Part print with two shaded views. Sizes in mm from the minimum x, y, z corner. A direction names the side the tool comes from. Coordinates: 2 decimals unless noted, no trailing zeros. Loops run counter-clockwise (first coordinate to the right, second up) from the corner with the lowest first, then second, coordinate; pieces in that order, holes last.
(1) Slice it at C-C (x = 3.5). Give the cut face in (y, z).
(2) Two-plate mould, pull along X, no slides. Class the marked faces 3, 4 and 5: pulls with the +X half, pulls with the -X half, needs draft (parallel to the pull), parting line crosses it, or undercut.
(3) Flat gauge pins, fed straight in: P1, Ø0.9, axis at x = 46, y = 36.5, coming from the +Z side; P2, Ø11.5, axis at x = 26.5, y = 22, coming from the +Z side. Where does each tip first touch, or does it go through?
(4) Slice it at A-A (z = 11.25). Give the cut face in (x, y), and give its area (3 significant figures).
(5) Slice it at D-D (z = 7.75). Give the cut face in (x, y).
(6) Tool access for the marked faces 1 and 2: list every direction of +Z, -Z, +X, -X, +Y, -Y with a clear straight run to the whole face (end or side of a thin tool).
(7) Wall check: L1, parallel to Y at x = 46.5, z = 15; L2, parallel to X at y = 2.5, z = 1.25; L3, parallel to Y at x = 43.5, z = 7.25. Give the ranges that are in metal, low to high.
(8) Slice it at B-B (y = 22). Give the cut face in (x, z), and give its area (3 significant figures).
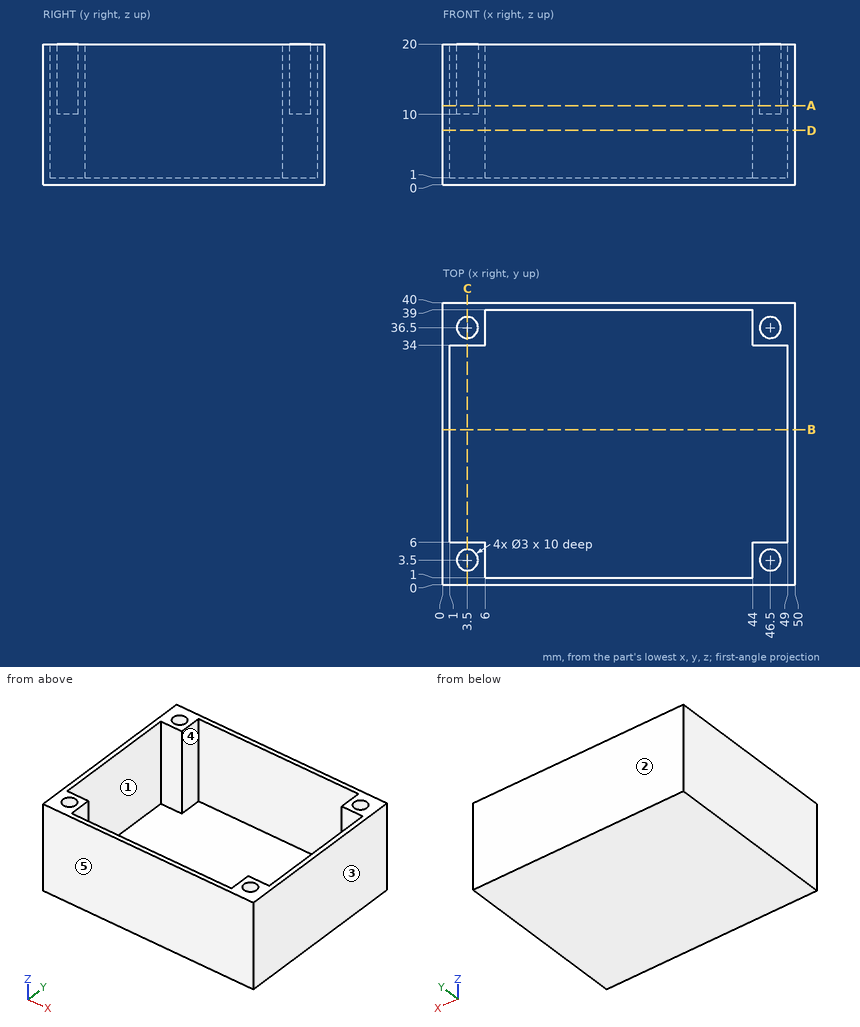
Response values:
1. outline: (0, 0) - (40, 0) - (40, 20) - (38, 20) - (38, 10) - (35, 10) - (35, 20) - (34, 20) - (34, 1) - (6, 1) - (6, 20) - (5, 20) - (5, 10) - (2, 10) - (2, 20) - (0, 20) - close
2. face 3: pulls with the +X half
2. face 4: undercut
2. face 5: needs draft
3. P1: stops at z = 10
3. P2: stops at z = 1
4. outline: (0, 0) - (50, 0) - (50, 40) - (0, 40) - close; hole (1, 6) - (6, 6) - (6, 1) - (44, 1) - (44, 6) - (49, 6) - (49, 34) - (44, 34) - (44, 39) - (6, 39) - (6, 34) - (1, 34) - close; hole circle Ø3 at (3.5, 3.5); hole circle Ø3 at (3.5, 36.5); hole circle Ø3 at (46.5, 3.5); hole circle Ø3 at (46.5, 36.5)
4. area: 248 mm2
5. outline: (0, 0) - (50, 0) - (50, 40) - (0, 40) - close; hole (1, 6) - (6, 6) - (6, 1) - (44, 1) - (44, 6) - (49, 6) - (49, 34) - (44, 34) - (44, 39) - (6, 39) - (6, 34) - (1, 34) - close
6. face 1: +Z
6. face 2: +Z, -Z, +X, -X, +Y
7. L1: y = 0 to 2, 5 to 6, 34 to 35, 38 to 40
7. L2: x = 0 to 6, 44 to 50
7. L3: y = 0 to 1, 39 to 40
8. outline: (0, 0) - (50, 0) - (50, 20) - (49, 20) - (49, 1) - (1, 1) - (1, 20) - (0, 20) - close
8. area: 88.0 mm2
